Could you check a few things on this model? Use its own coordinates, in mm. A direction names the side the tool comes from. Coordinates: 2 decimals unless noted, no trailing zeros. Loops run counter-clockwise (first coordinate to the right, second up) from the corner with the lowest first, then second, coordinate; pieces in that order, holes last. Notation, with made-up numbers: M 4.5,81 L 35.5,81 A33 cw 35.5,111 Z; hole C 74,60 d8. An arc over 180 degrees is marked long. Write each question's results on one line, items separated by ' | '.
```python
from build123d import *

# Parameters (mm, degrees)
BASE_FLANGE1_DEPTH = 0.625
FILLET1_RADIUS     = 0.625
FILLET1_LENGTH     = 0.25
HOLE1_START        = -1.5
HOLE1_OUTLINE_R    = 0.175
HOLE1_DEPTH        = 0.25


# Read off the part's stored shape, not the designer's step: Hole1
# Sheet-metal steps are written as plain solids
with BuildPart() as part:
    # Sketch1 → Base-Flange1 (new, symmetric)
    with BuildSketch(Plane(origin=(0, 0, 0), x_dir=(0, 0, -1), z_dir=(1, 0, 0))):
        with BuildLine():
            Line((12, 0), (0.15, 0))
            ThreePointArc((0.15, 0), (0.043933983, -0.043933983), (0, -0.15))
            Line((0, -0.15), (0, -1.1))
            ThreePointArc((0, -1.1), (-0.117157288, -1.382842712), (-0.4, -1.5))
            Line((-0.4, -1.5), (-1.5, -1.5))
            Line((-1.5, -1.5), (-1.5, -1.25))
            Line((-1.5, -1.25), (-0.4, -1.25))
            ThreePointArc((-0.4, -1.25), (-0.293933983, -1.206066017), (-0.25, -1.1))
            Line((-0.25, -1.1), (-0.25, -0.15))
            ThreePointArc((-0.25, -0.15), (-0.132842712, 0.132842712), (0.15, 0.25))
            Line((0.15, 0.25), (12, 0.25))
            Line((12, 0.25), (12, 0))
        make_face()
    extrude(amount=BASE_FLANGE1_DEPTH, both=True)

    # Fillet1: full round fillet: the end face becomes a half cylinder, R = half its width
    fillet1_face = Plane((0, -1.375, 1.5), x_dir=(0, -1, 0), z_dir=(0, 0, 1))  # on the end face: x along it, z out of the body
    fillet1_slab = fillet1_face.offset(-FILLET1_RADIUS / 2) * Box(FILLET1_LENGTH, 2 * FILLET1_RADIUS, FILLET1_RADIUS, mode=Mode.PRIVATE)  # the body's end, R deep
    fillet1_round = Plane((0, -1.375, 0.875), x_dir=(0, 0, 1), z_dir=(0, -1, 0)) * Cylinder(FILLET1_RADIUS, FILLET1_LENGTH, mode=Mode.PRIVATE)  # its axis R under the face
    add(fillet1_slab - fillet1_round, mode=Mode.SUBTRACT)

    # Hole1 outline → Hole1 (cut)
    with BuildSketch(Plane(origin=(0, 0, 0), x_dir=(1, 0, 0), z_dir=(0, 1, 0)).offset(HOLE1_START)):
        with Locations((0.001471382, -0.886025874)):
            Circle(HOLE1_OUTLINE_R)
    extrude(amount=HOLE1_DEPTH, mode=Mode.SUBTRACT)


solid = part.part
```
(1) Imagine slicing it at B-B, the plane x = -0.5. List the corners of the cut face in (y, z) for me.
Reported:
outline: M -1.5,0.4 A0.4 ccw -1.1,0 L -0.15,0 A0.15 cw 0,-0.15 L 0,-12 L 0.25,-12 L 0.25,-0.15 A0.4 ccw -0.15,0.25 L -1.1,0.25 A0.15 cw -1.25,0.4 L -1.25,1.25 L -1.5,1.25 Z
(2) Imagine slicing it at C-C, the plane z = -2. List the corners of the cut face in (x, y) for me (3 decimals).
Reported:
outline: M -0.625,0 L 0.625,0 L 0.625,0.25 L -0.625,0.25 Z
(3) Please list where this line runs through material, in increasing order: probe 1 along Z at (x, y) = (-0.1, -0.35). Write a range as from..to.
Reported:
probe 1: z = 0..0.25
(4) Imagine slicing it at A-A, the plane x = 0. List the corners of the cut face in (y, z) for me.
Reported:
outline: M -1.5,0.4 A0.4 ccw -1.1,0 L -0.15,0 A0.15 cw 0,-0.15 L 0,-12 L 0.25,-12 L 0.25,-0.15 A0.4 ccw -0.15,0.25 L -1.1,0.25 A0.15 cw -1.25,0.4 L -1.25,0.71 L -1.5,0.71 Z; M -1.5,1.06 L -1.25,1.06 L -1.25,1.5 L -1.5,1.5 Z
(5) Which directions (+Z, -Z, +X, -X, +Y, -Y) give clear straight access to the entire face, cutting with the end or side of a thin tool? Please do faces 1 (the flat face through (0, -0.6, 0)), 2 (the flat face through (0, -0.6, 0.25)), 3 (the flat face through (0, 0.25, -6)).
Reported:
face 1: -Z, +X, -X, -Y | face 2: +Z, +X, -X, +Y | face 3: +Z, -Z, +X, -X, +Y
